from build123d import *

# Parameters (mm, degrees)
F0_W      = 14.3
F0_H      = 19
F0_R      = 1
F0_W_2    = 0.8
F0_H_2    = 1.8
F0_W_3    = 1.3
F0_H_3    = 3
F0_W_4    = 2.5
F0_H_4    = 1.58
F0_W_5    = 1.8
F0_H_5    = 0.8
F0_R_2    = 1.5
F1_DEPTH  = 1.6
F2_DEPTH  = 0.75
F3_DEPTH  = 0.9
F4_DEPTH  = 0.5
F5_DEPTH  = 1.04
F6_DEPTH  = 1.8
F7_SIZE2  = 0.9
F7_SIZE   = 0.9
F8_W      = 0.7
F8_H      = 0.7
F9_DEPTH  = 14.4
F8_W_2    = 12.86
F8_H_2    = 2.54
F10_DEPTH = 11.4


with BuildPart() as f1:
    # F0 (on Top) → F1 (new body)
    with BuildSketch(Plane.XY):
        Rectangle(F0_W, F0_H)
        with Locations((-5.08, -7.9)):
            Circle(F0_R, mode=Mode.SUBTRACT)
        with Locations((-2.54, -7.9)):
            Circle(F0_R, mode=Mode.SUBTRACT)
        with BuildLine():
            ThreePointArc((0, -6.9), (1, -7.9), (0, -8.9))
            ThreePointArc((0, -8.9), (-1, -7.9), (0, -6.9))
        make_face(mode=Mode.SUBTRACT)
        with Locations((-5.95, -4.4)):
            Rectangle(F0_W_2, F0_H_2, mode=Mode.SUBTRACT)
        with Locations((-4.35, -4.4)):
            Rectangle(F0_W_2, F0_H_2, mode=Mode.SUBTRACT)
        with Locations((-2.75, -4.4)):
            Rectangle(F0_W_2, F0_H_2, mode=Mode.SUBTRACT)
        with Locations((-1.15, -4.4)):
            Rectangle(F0_W_2, F0_H_2, mode=Mode.SUBTRACT)
        with Locations((2.54, -7.9)):
            Circle(F0_R, mode=Mode.SUBTRACT)
        with Locations((5.08, -7.9)):
            Circle(F0_R, mode=Mode.SUBTRACT)
        with Locations((0.45, -4.4)):
            Rectangle(F0_W_2, F0_H_2, mode=Mode.SUBTRACT)
        with Locations((3.2, -4.4)):
            Rectangle(F0_W_3, F0_H_3, mode=Mode.SUBTRACT)
        with Locations((5.95, -4.4)):
            Rectangle(F0_W_2, F0_H_2, mode=Mode.SUBTRACT)
        with Locations((0, 1.71)):
            Rectangle(F0_W_4, F0_H_4, mode=Mode.SUBTRACT)
        with Locations((0, 4.1)):
            Rectangle(F0_W_5, F0_H_5, mode=Mode.SUBTRACT)
        with Locations((-4.15, 6)):
            Circle(F0_R_2, mode=Mode.SUBTRACT)
        with Locations((0, 5.4)):
            Rectangle(F0_W_5, F0_H_5, mode=Mode.SUBTRACT)
        with Locations((4.15, 6)):
            Circle(F0_R_2, mode=Mode.SUBTRACT)
        with Locations((0, 1.71)):
            Rectangle(F0_W_4, F0_H_4)
        with Locations((5.95, -4.4)):
            Rectangle(F0_W_2, F0_H_2)
        with Locations((3.2, -4.4)):
            Rectangle(F0_W_3, F0_H_3)
        with Locations((0.45, -4.4)):
            Rectangle(F0_W_2, F0_H_2)
        with Locations((-1.15, -4.4)):
            Rectangle(F0_W_2, F0_H_2)
        with Locations((-2.75, -4.4)):
            Rectangle(F0_W_2, F0_H_2)
        with Locations((-4.35, -4.4)):
            Rectangle(F0_W_2, F0_H_2)
        with Locations((-5.95, -4.4)):
            Rectangle(F0_W_2, F0_H_2)
        with Locations((0, 4.1)):
            Rectangle(F0_W_5, F0_H_5)
        with Locations((0, 5.4)):
            Rectangle(F0_W_5, F0_H_5)
        with Locations((-5.08, -7.9)):
            Circle(F0_R)
        with Locations((-2.54, -7.9)):
            Circle(F0_R)
        with BuildLine():
            ThreePointArc((0, -6.9), (-1, -7.9), (0, -8.9))
            ThreePointArc((0, -8.9), (1, -7.9), (0, -6.9))
        make_face()
        with Locations((2.54, -7.9)):
            Circle(F0_R)
        with Locations((5.08, -7.9)):
            Circle(F0_R)
    extrude(amount=-F1_DEPTH)

    # F0 (on Top) → F2 (join)
    with BuildSketch(Plane.XY):
        with Locations((0, 1.71)):
            Rectangle(F0_W_4, F0_H_4)
    extrude(amount=F2_DEPTH)

    # F0 (on Top) → F3 (join)
    with BuildSketch(Plane.XY):
        with Locations((0, 5.4)):
            Rectangle(F0_W_5, F0_H_5)
        with Locations((5.95, -4.4)):
            Rectangle(F0_W_2, F0_H_2)
        with Locations((0.45, -4.4)):
            Rectangle(F0_W_2, F0_H_2)
        with Locations((-1.15, -4.4)):
            Rectangle(F0_W_2, F0_H_2)
    extrude(amount=F3_DEPTH)

    # F0 (on Top) → F4 (join)
    with BuildSketch(Plane.XY):
        with Locations((0, 4.1)):
            Rectangle(F0_W_5, F0_H_5)
        with Locations((-2.75, -4.4)):
            Rectangle(F0_W_2, F0_H_2)
        with Locations((-4.35, -4.4)):
            Rectangle(F0_W_2, F0_H_2)
        with Locations((-5.95, -4.4)):
            Rectangle(F0_W_2, F0_H_2)
    extrude(amount=F4_DEPTH)

    # F0 (on Top) → F5 (join)
    with BuildSketch(Plane.XY):
        with Locations((3.2, -4.4)):
            Rectangle(F0_W_3, F0_H_3)
    extrude(amount=F5_DEPTH)

    # F0 (on Top) → F6 (join)
    with BuildSketch(Plane.XY):
        with Locations((-5.08, -7.9)):
            Circle(F0_R)
        with Locations((-2.54, -7.9)):
            Circle(F0_R)
        with BuildLine():
            ThreePointArc((0, -6.9), (-1, -7.9), (0, -8.9))
            ThreePointArc((0, -8.9), (1, -7.9), (0, -6.9))
        make_face()
        with Locations((2.54, -7.9)):
            Circle(F0_R)
        with Locations((5.08, -7.9)):
            Circle(F0_R)
    extrude(amount=F6_DEPTH)

    # F7
    f7_edges = [f1.edges().sort_by_distance(p)[0] for p in [
        (-6.08, -7.9, 1.8),
        (-3.54, -7.9, 1.8),
        (0, -6.9, 1.8),
        (1.54, -7.9, 1.8),
        (4.08, -7.9, 1.8),
    ]]
    chamfer(f7_edges, length=F7_SIZE, length2=F7_SIZE2)

    # F8 (on face) → F9 (join)
    with BuildSketch(Plane(origin=(0, 0, -1.6), x_dir=(1, 0, 0), z_dir=(0, 0, -1))):
        with Locations((-5.08, 7.9)):
            Rectangle(F8_W, F8_H)
        with Locations((-2.54, 7.9)):
            Rectangle(F8_W, F8_H)
        with Locations((0, 7.9)):
            Rectangle(F8_W, F8_H)
        with Locations((2.54, 7.9)):
            Rectangle(F8_W, F8_H)
        with Locations((5.08, 7.9)):
            Rectangle(F8_W, F8_H)
    extrude(amount=F9_DEPTH)

    # F8 (on face) → F10 (join)
    with BuildSketch(Plane(origin=(0, 0, -1.6), x_dir=(1, 0, 0), z_dir=(0, 0, -1))):
        with Locations((0, 7.9)):
            Rectangle(F8_W_2, F8_H_2)
        with Locations((-5.08, 7.9)):
            Rectangle(F8_W, F8_H, mode=Mode.SUBTRACT)
        with Locations((-2.54, 7.9)):
            Rectangle(F8_W, F8_H, mode=Mode.SUBTRACT)
        with Locations((0, 7.9)):
            Rectangle(F8_W, F8_H, mode=Mode.SUBTRACT)
        with Locations((2.54, 7.9)):
            Rectangle(F8_W, F8_H, mode=Mode.SUBTRACT)
        with Locations((5.08, 7.9)):
            Rectangle(F8_W, F8_H, mode=Mode.SUBTRACT)
    extrude(amount=F10_DEPTH)


solid = f1.part
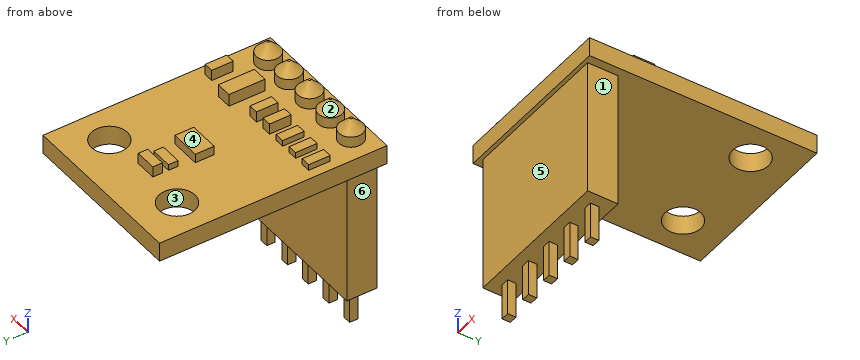
Build history of the part. All positions in model axes, mm. Face numbers are marked on the shaded views. A direction names the side the tool comes from. Give positions to 0.01 mm unless a question says otherwise; leave off trailing zeros. Order: outer loops, then holes, each group sorted by start corner. A loop starts at its lowest first (then second) coordinate and runs counter-clockwise, first axis right, second up. Notation, with made-up numbers: M 75.5,46 L 134.5,46 A24 ccw 134.5,83 Z; hole C 87,-17 d9. An arc over 180 degrees is marked long. Put each result on its own line as item: value.
Item 1: Slice it at A-A, the plane y = 2.25. Write the cut outline in (x, z).
From the geometry:
outline: M -7.15,-1.6 L 7.15,-1.6 L 7.15,0 L 1.25,0 L 1.25,0.75 L -1.25,0.75 L -1.25,0 L -7.15,0 Z
Item 2: Slice it at C-C, the plane y = -0.5. Write the cut outline in (x, z), plus the area to 3 significant figures.
From the geometry:
outline: M -7.15,-1.6 L 7.15,-1.6 L 7.15,0 L -7.15,0 Z
area: 22.9 mm2
Item 3: Slice it at B-B, the plane z = -12.5. Write the cut outline in (x, y), plus the area to 3 significant figures.
From the geometry:
outline: M -6.43,-9.17 L 6.43,-9.17 L 6.43,-6.63 L -6.43,-6.63 Z
area: 32.7 mm2
Item 4: 3-axis set-ups, long thin cutter, end or side, ignore diameter. For the marked faces 4, 5 and 6: which of +Z, -Z, +X, -X, +Y, -Y reach the whole face in a straight line?
From the geometry:
face 4: +Z, +X, -X
face 5: -Z, +X, -X, -Y
face 6: -Z, -X, +Y, -Y
Item 5: Probe line 1 (Y direction, x = 4.15, z = -0.5); line 2 (Z direction, x = 3.25, y = 8.5); line 3 (Y direction, x = -4.5, z = -2.25). List the from-to ranges inside material, lowest first. Write a range as [from, to].
From the geometry:
line 1: y = [-9.5, 4.5], [7.5, 9.5]
line 2: z = [-1.6, 0]
line 3: y = [-9.17, -6.63]
Item 6: Flat gauge pins, fed straight in: pin 1 Ø6 at (x, y) = (-3, 6.5) entering from +Z; pin 2 Ø0.6 at (x, z) = (2.5, -14) entering from +Y; pin 3 Ø0.6 at (x, z) = (-1.5, 0.5) entering from -Y. Where does each tip first touch, or does it go through?
From the geometry:
pin 1: stops at z = 0.9
pin 2: stops at y = -7.55
pin 3: stops at y = -8.57
Item 7: Two-plate mould, pull along Y, no slides. Class the marked faces 1, 2 and 3: +Y half, -Y half, draft (parallel to the pull), parting line (faces both ways), or undercut.
From the geometry:
face 1: draft
face 2: parting line
face 3: undercut
